Read the model definition and answer for the solid it produces. Units are mm, in the model's axes. Face numbers are marked on the shaded views. A direction names the side the tool comes from. Give positions to 0.01 mm unless a question says otherwise; leave off trailing zeros. Loops run counter-clockwise (first coordinate to the right, second up) from the corner with the lowest first, then second, coordinate; pieces in that order, holes last. Notation, with made-up numbers: (71.25, 27.25) - (122.25, 27.25) arc R23 ccw to (122.25, 64.25) - close; hole circle Ø9 at (70, 36.25). An arc over 180 degrees is marked (long way). Use a Markdown table: item, result. Add a question column.
Item 1: A cutting plane is placed at B-B (z = 8). Determine the outline of the cut face in (x, y), plus the area to 3 significant figures.
Item 2: Consider probe 1 along X at (y, z) = (0, 4); probe 2 along X at (y, z) = (0, 2). Determine where each line is inside the solid, lowest interval first. Write a range as [from, to].
Item 3: Each of these flat-tipped pins is pushed along its axis until it touches: P1, Ø2, axis at x = 7.5, y = -1, coming from the -Z side; P2, Ø0.5, axis at x = 0, y = 1, coming from the +Z side; P3, Ø1.2, axis at x = 6.5, y = -0.5, coming from the +Z side. Where does it stop, or does it pass through?
Item 4: A cutting plane is placed at C-C (x = 6.5). Determine the outline of the cut face in (y, z), plus the area to 3 significant figures.
Item 5: For a pull along X with two mould halves and no side action, classify the marked faces 3, 4, 5 and 6 as +X half, -X half, draft (parallel to the pull), parting line (faces both ways), or undercut.
Item 6: A cutting plane is placed at D-D (z = 2). Determine the outline of the cut face in (x, y).
Item 7: A cutting plane is placed at A-A (z = 4.5). Determine the outline of the cut face in (x, y), plus the area to 3 significant figures.
Item 8: Which of the six approach directions +Z, -Z, +X, -X, +Y, -Y give full straight-line access (tool end or side, diameter ignored) to the marked faces 1 and 2?
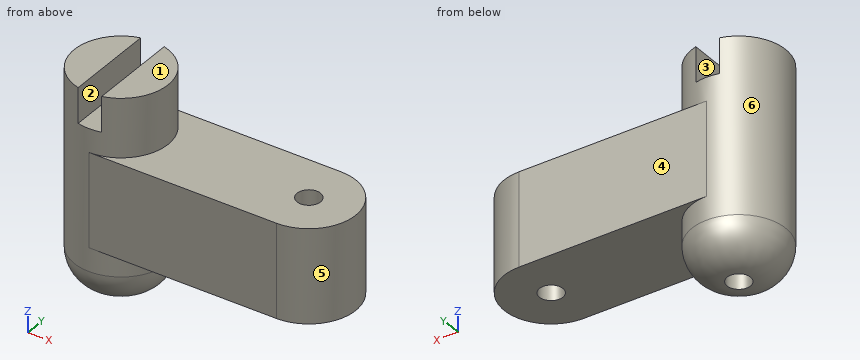
from build123d import *

# Parameters (mm, degrees)
SKETCH_1_R          = 2
SKETCH_1_R_2        = 0.5
EXTRUDE_1_DEPTH     = 9
SKETCH_2_W          = 1
SKETCH_2_H          = 4.164709902
CUT_EXTRUDE_1_DEPTH = 1.5
FILLET_2_R          = 1.5
SKETCH_3_W          = 8
SKETCH_3_H          = 4
EXTRUDE_2_DEPTH     = 2
SKETCH_4_R          = 2
SKETCH_4_R_2        = 0.5
EXTRUDE_3_DEPTH     = 4
SKETCH_5_R          = 0.5
CUT_EXTRUDE_2_DEPTH = 4
SKETCH_6_R          = 0.5
CUT_EXTRUDE_3_DEPTH = 14.601470509


with BuildPart() as part:
    # 草图1 → 凸台-拉伸1 (new body)
    with BuildSketch(Plane.XY):
        Circle(SKETCH_1_R)
        Circle(SKETCH_1_R_2, mode=Mode.SUBTRACT)
    extrude(amount=EXTRUDE_1_DEPTH)

    # 草图2 → 切除-拉伸1 (cut)
    with BuildSketch(Plane.XY.offset(9)):
        Rectangle(SKETCH_2_W, SKETCH_2_H)
    extrude(amount=-CUT_EXTRUDE_1_DEPTH, mode=Mode.SUBTRACT)

    # 圆角2
    fillet_2_edges = [part.edges().sort_by_distance(p)[0] for p in [
        (-2, 0, 0),
    ]]
    fillet(fillet_2_edges, radius=FILLET_2_R - 0.0001)  # a hair under: the kernel refuses the full size

    # 草图3 → 凸台-拉伸2 (add, symmetric)
    with BuildSketch(Plane(origin=(0, 0, 0), x_dir=(1, 0, 0), z_dir=(0, 1, 0))):
        with Locations((4, -4.5)):
            Rectangle(SKETCH_3_W, SKETCH_3_H)
    extrude(amount=EXTRUDE_2_DEPTH, both=True)

    # 草图4 → 凸台-拉伸3 (add)
    with BuildSketch(Plane(origin=(0, 0, 2.5), x_dir=(-1, 0, 0), z_dir=(0, 0, -1))):
        with Locations((-8, 0)):
            Circle(SKETCH_4_R)
        with Locations((-8, 0)):
            Circle(SKETCH_4_R_2, mode=Mode.SUBTRACT)
    extrude(amount=-EXTRUDE_3_DEPTH)

    # 草图5 → 切除-拉伸2 (cut)
    with BuildSketch(Plane(origin=(0, 0, 2.5), x_dir=(-1, 0, 0), z_dir=(0, 0, -1))):
        with Locations((-8, 0)):
            Circle(SKETCH_5_R)
    extrude(amount=-CUT_EXTRUDE_2_DEPTH, mode=Mode.SUBTRACT)

    # 草图6 → 切除-拉伸3 (cut, through all)
    with BuildSketch(Plane.XY.offset(9)):
        Circle(SKETCH_6_R)
    extrude(amount=-CUT_EXTRUDE_3_DEPTH, mode=Mode.SUBTRACT)


solid = part.part
Geometry says:
| question | item | result |
|---|---|---|
| 1 | outline | (-0.5, -1.94) - (-0.5, 1.94) arc R2 ccw to start; (0.5, -1.94) arc R2 ccw to (0.5, 1.94) - close |
| 1 | area | 8.61 mm² |
| 2 | probe 1 | [-2, -0.5], [0.5, 7.5], [8.5, 10] |
| 2 | probe 2 | [-2, -0.5], [0.5, 2] |
| 3 | P1 | z = 2.5 |
| 3 | P2 | z = 7.5 |
| 3 | P3 | z = 6.5 |
| 4 | outline | (-2, 2.5) - (2, 2.5) - (2, 6.5) - (-2, 6.5) - close |
| 4 | area | 16.0 mm² |
| 5 | face 3 | undercut |
| 5 | face 4 | draft |
| 5 | face 5 | +X half |
| 5 | face 6 | parting line |
| 6 | outline | circle Ø4 at (0, 0); hole circle Ø1 at (0, 0) |
| 7 | outline | (0, -2) - (8, -2) arc R2 ccw to (8, 2) - (0, 2) arc R2 ccw to start; hole circle Ø1 at (0, 0); hole circle Ø1 at (8, 0) |
| 7 | area | 43.0 mm² |
| 8 | face 1 | +Z, +X, -X, +Y, -Y |
| 8 | face 2 | +Z, +Y, -Y |
